Source: CAD feature listing. Evaluate the final solid. Frame: model axes, mm. A direction names the side the tool comes from. Give positions to 0.01 mm unless a question says otherwise; leave off trailing zeros. Loops run counter-clockwise (first coordinate to the right, second up) from the corner with the lowest first, then second, coordinate; pieces in that order, holes last. Notation, with made-up numbers: (81.5, -20.75) - (130.5, -20.75) arc R14 cw to (130.5, 0.25) - close; hole circle Ø1 at (-4, -29). An arc over 180 degrees is marked (long way). Put each result on its own line as item: value.
```python
from build123d import *

# Parameters (mm, degrees)
SKETCH1_W           = 23
SKETCH1_H           = 23
BOSS_EXTRUDE1_DEPTH = 2.4
FILLET1_R           = 2
SKETCH2_R           = 2
BOSS_EXTRUDE2_DEPTH = 2.4
FILLET2_R           = 2


with BuildPart() as part:
    # Sketch1 → Boss-Extrude1 (new body)
    with BuildSketch(Plane(origin=(0, 0, 0), x_dir=(1, 0, 0), z_dir=(0, 1, 0))):
        Rectangle(SKETCH1_W, SKETCH1_H)
    extrude(amount=BOSS_EXTRUDE1_DEPTH)

    # Fillet1
    fillet1_edges = [part.edges().sort_by_distance(p)[0] for p in [
        (-11.5, 1.2, -11.5),
        (11.5, 1.2, -11.5),
    ]]
    fillet(fillet1_edges, radius=FILLET1_R)

    # Sketch2 → Boss-Extrude2 (add)
    with BuildSketch(Plane(origin=(0, 2.4, 0), x_dir=(1, 0, 0), z_dir=(0, 1, 0))):
        with BuildLine():
            Line((-3, -11.5), (-3, -16.5))
            ThreePointArc((-3, -16.5), (0, -19.5), (3, -16.5))
            Line((3, -16.5), (3, -11.5))
            Line((3, -11.5), (-3, -11.5))
        make_face()
        with Locations((0, -16.5)):
            Circle(SKETCH2_R, mode=Mode.SUBTRACT)
    extrude(amount=-BOSS_EXTRUDE2_DEPTH)

    # Fillet2
    fillet2_edges = [part.edges().sort_by_distance(p)[0] for p in [
        (3, 1.2, 11.5),
        (-3, 1.2, 11.5),
    ]]
    fillet(fillet2_edges, radius=FILLET2_R)


solid = part.part
```
1) Section query A-A, the plane x = 0. Output: boundary loops of the cut face in (y, z).
Check result:
outline: (0, -11.5) - (2.4, -11.5) - (2.4, 14.5) - (0, 14.5) - close; (0, 18.5) - (2.4, 18.5) - (2.4, 19.5) - (0, 19.5) - close
2) Access query for faces 4 (the flat face through (-8, 1, 11.5)), 5 (the flat face through (0, 1, -11.5)), 6 (the flat face through (8, 1, 11.5)). Directions: +Z, -Z, +X, -X, +Y, -Y. A direction counts if a zero-diameter tool reaches every point of the face in a straight line with its end or side. Return the directions, or none.
Check result:
face 4: +Z, -X, +Y, -Y
face 5: -Z, +X, -X, +Y, -Y
face 6: +Z, +X, +Y, -Y
3) Section query B-B, the plane y = 0.95. Output: boundary loops of the cut face in (x, z), plus the area to 3 significant figures.
Check result:
outline: (-11.5, -9.5) arc R2 ccw to (-9.5, -11.5) - (9.5, -11.5) arc R2 ccw to (11.5, -9.5) - (11.5, 11.5) - (5, 11.5) arc R2 cw to (3, 13.5) - (3, 16.5) arc R3 ccw to (-3, 16.5) - (-3, 13.5) arc R2 cw to (-5, 11.5) - (-11.5, 11.5) - close; hole circle Ø4 at (0, 16.5)
area: 561 mm²
4) Mould query, pull axis Z, two halves, no side actions, for faces 1 (the flat face through (0, 2.4, 0)), 2 (the cylindrical face through (-0.26, 1.217, 14.517)), 3 (the cylindrical face through (-3.6, 1.18, 12.07)). Classes: pulls with the +Z half, pulls with the -Z half, needs draft (parallel to the pull), parting line crosses it, or undercut.
Check result:
face 1: needs draft
face 2: undercut
face 3: pulls with the +Z half
5) Section query C-C, the plane x = -6.5. Output: boundary loops of the cut face in (y, z).
Check result:
outline: (0, -11.5) - (2.4, -11.5) - (2.4, 11.5) - (0, 11.5) - close
6) Material intervals for line 1 along X through (y, z) = (1.15, 16.5); line 2 along Z through (x, y) = (0, 1.3); line 3 along Z through (x, y) = (7.5, 1.45), sorted ascending. Write a range as [from, to].
Check result:
line 1: [-3, -2], [2, 3]
line 2: [-11.5, 14.5], [18.5, 19.5]
line 3: [-11.5, 11.5]
7) Pin query (flat end, axial travel): P1, Ø0.7, axis at y = 1.5, z = 15, coming from the -X side; P2, Ø1.2, axis at x = 8.5, y = 1.5, coming from the +Z side; P3, Ø1.2, axis at y = 1, z = 15.5, coming from the +X side; P4, Ø3, axis at x = 0, z = 16.5, coming from the -Y side. Return the tip coordinate at first contact, or that it passes through.
Check result:
P1: x = -3
P2: z = 11.5
P3: x = 3
P4: through
8) Section query D-D, the plane z = 12. Output: boundary loops of the cut face in (x, y).
Check result:
outline: (-3.68, 0) - (3.68, 0) - (3.68, 2.4) - (-3.68, 2.4) - close
